The listing builds one solid part. Answer for the finished solid, in the listing's coordinates (mm). Round coordinates to 2 decimals unless told otherwise and drop trailing zeros. Order: outer loops, then holes, each group sorted by start corner. A loop starts at its lowest first (then second) coordinate and runs counter-clockwise, first axis right, second up. Notation, with made-up numbers: (53.25, 8) -> (93.25, 8) arc R10 cw to (93.25, 14) -> close; hole circle Ø4 at (-17, 58). An arc over 180 degrees is marked (long way). Return JSON: item names as keys, results as strings. Group by question number.
(1) The part is cut by section B-B (y = 312.5). Determine the outline of the cut face in (x, z).
(2) The part is cut by section C-C (z = 34). Determine the outline of the cut face in (x, y), plus the area to 3 significant figures.
(3) The part is cut by section A-A (x = 3.25). Determine the outline of the cut face in (y, z), plus the area to 3 significant figures.
(4) Consider line 1 (Z direction, x = 15.75, y = -171.5); line 2 (Z direction, x = 11.5, y = 291). Determine where each line is inside the solid, lowest interval first. Write a range as [from, to].
from build123d import *

# Parameters (mm, degrees)
F1_DEPTH = 19.05
F3_DEPTH = 25.4
F4_DEPTH = 3.175


with BuildPart() as f1:
    # F0 (on Right) → F1 (new body)
    with BuildSketch(Plane.YZ):
        with BuildLine():
            ThreePointArc((482.6, 127), (467.7210244843, 162.9210244843), (431.8, 177.8))
            Line((431.8, 177.8), (-482.6, -152.4))
            ThreePointArc((-482.6, -152.4), (-475.1605122421, -170.3605122421), (-457.2, -177.8))
            Line((-457.2, -177.8), (431.8, -177.8))
            ThreePointArc((431.8, -177.8), (467.7210244843, -162.9210244843), (482.6, -127))
            Line((482.6, -127), (482.6, 127))
        make_face()
    extrude(amount=F1_DEPTH)

    # F2 (on face) → F3 (cut)
    with BuildSketch(Plane.YZ.offset(19.05)):
        with BuildLine():
            Line((461.4467891453, 168.2517623063), (433.3557372898, 158.1077713585))
            Line((433.3557372898, 158.1077713585), (433.3557372898, -158.75))
            Line((433.3557372898, -158.75), (471.4557372898, -158.75))
            ThreePointArc((471.4557372898, -158.75), (479.733033778, -143.8245140446), (482.6, -127))
            Line((482.6, -127), (482.6, 127))
            ThreePointArc((482.6, 127), (477.0034118656, 150.1795503776), (461.4467891453, 168.2517623063))
        make_face()
        with BuildLine():
            Line((431.8, 177.8), (-25.4, 12.7))
            Line((-25.4, 12.7), (-18.929772965, -5.2175517891))
            Line((-18.929772965, -5.2175517891), (433.3557372898, 158.1077713585))
            Line((433.3557372898, 158.1077713585), (461.4467891453, 168.2517623063))
            ThreePointArc((461.4467891453, 168.2517623063), (447.3732218061, 175.3540563198), (431.8, 177.8))
        make_face()
        with BuildLine():
            Line((-18.929772965, -5.2175517891), (-25.4, 12.7))
            Line((-25.4, 12.7), (-482.6, -152.4))
            ThreePointArc((-482.6, -152.4), (-480.7436230259, -161.931936572), (-475.4458413533, -170.0705764849))
            Line((-475.4458413533, -170.0705764849), (-444.0965526259, -158.75))
            Line((-444.0965526259, -158.75), (-18.929772965, -5.2175517891))
        make_face()
        with BuildLine():
            Line((-12.7, -158.75), (-444.0965526259, -158.75))
            Line((-444.0965526259, -158.75), (-475.4458413533, -170.0705764849))
            ThreePointArc((-475.4458413533, -170.0705764849), (-467.1077585074, -175.7879524832), (-457.2, -177.8))
            Line((-457.2, -177.8), (-12.7, -177.8))
            Line((-12.7, -177.8), (-12.7, -158.75))
        make_face()
        with BuildLine():
            Line((471.4557372898, -158.75), (433.3557372898, -158.75))
            Line((433.3557372898, -158.75), (-12.7, -158.75))
            Line((-12.7, -158.75), (-12.7, -177.8))
            Line((-12.7, -177.8), (431.8, -177.8))
            ThreePointArc((431.8, -177.8), (453.7970452561, -172.7905011984), (471.4557372898, -158.75))
        make_face()
    extrude(amount=-F3_DEPTH, mode=Mode.SUBTRACT)

    # F4 (cut): a face of the model
    f4_faces = [f1.faces().sort_by_distance(p)[0] for p in [
        (9.525, -5.370407668, -0.3211143208),
    ]]
    extrude(f4_faces, amount=-F4_DEPTH, mode=Mode.SUBTRACT)


solid = f1.part
Answer below:
{
 "1": {"outline": "(0, -158.75) -> (19.05, -158.75) -> (19.05, 111.09) -> (0, 111.09) -> close"},
 "2": {"outline": "(0, 99.02) -> (19.05, 99.02) -> (19.05, 433.36) -> (0, 433.36) -> close", "area": "6,370 mm²"},
 "3": {"outline": "(-434.75, -158.75) -> (433.36, -158.75) -> (433.36, 154.73) -> close", "area": "136,000 mm²"},
 "4": {"line 1": "z = [-158.75, -63.69]", "line 2": "z = [-158.75, 103.33]"}
}
